For this review, take the finished solid that the model builds, in its own axes (mm). Give positions to 0.01 mm unless a question says otherwise; leave off trailing zeros. Order: outer loops, then holes, each group sorted by start corner. A loop starts at its lowest first (then second) coordinate and runs counter-clockwise, first axis right, second up.
from build123d import *

# Parameters (mm, degrees)
SKETCH1_W           = 48.2
SKETCH1_H           = 18
SKETCH1_R           = 0.6
BOSS_EXTRUDE2_DEPTH = 1.6
SKETCH2_R           = 0.45
CUT_EXTRUDE2_DEPTH  = 1.6
LPATTERN1_COUNT     = 17
LPATTERN1_PITCH     = 2.54
SKETCH3_R           = 0.5
CUT_EXTRUDE4_DEPTH  = 1.6


with BuildPart() as part:
    # Sketch1 → Boss-Extrude2 (new body)
    with BuildSketch(Plane(origin=(0, 0, 0), x_dir=(1, 0, 0), z_dir=(0, 1, 0))):
        with Locations((20.32, 7.62)):
            Rectangle(SKETCH1_W, SKETCH1_H)
        with Locations((-2.54, 0)):
            Circle(SKETCH1_R, mode=Mode.SUBTRACT)
        with Locations((-2.54, 15.24)):
            Circle(SKETCH1_R, mode=Mode.SUBTRACT)
        with Locations((43.18, 15.24)):
            Circle(SKETCH1_R, mode=Mode.SUBTRACT)
        with Locations((43.18, 0)):
            Circle(SKETCH1_R, mode=Mode.SUBTRACT)
    extrude(amount=BOSS_EXTRUDE2_DEPTH)

    # Sketch2 → Cut-Extrude2 (cut)
    with BuildSketch(Plane(origin=(0, 0, 0), x_dir=(1, 0, 0), z_dir=(0, 1, 0))):
        Circle(SKETCH2_R)
        with Locations((0, 15.24)):
            Circle(SKETCH2_R)
    cut_extrude2 = extrude(amount=CUT_EXTRUDE2_DEPTH, mode=Mode.SUBTRACT)

    # LPattern1: Cut-Extrude2 ×17
    with Locations(*[(i * LPATTERN1_PITCH, 0, 0) for i in range(1, LPATTERN1_COUNT)]):
        add(cut_extrude2, mode=Mode.SUBTRACT)

    # Sketch3 → Cut-Extrude4 (cut)
    with BuildSketch(Plane(origin=(0, 0, 0), x_dir=(1, 0, 0), z_dir=(0, 1, 0))):
        with Locations((1.27, 12.7)):
            Circle(SKETCH3_R)
        with Locations((-1.27, 12.7)):
            Circle(SKETCH3_R)
        with Locations((-1.27, 10.16)):
            Circle(SKETCH3_R)
        with Locations((3.81, 12.7)):
            Circle(SKETCH3_R)
        with Locations((3.81, 10.16)):
            Circle(SKETCH3_R)
        with Locations((1.27, 10.16)):
            Circle(SKETCH3_R)
    extrude(amount=CUT_EXTRUDE4_DEPTH, mode=Mode.SUBTRACT)


solid = part.part
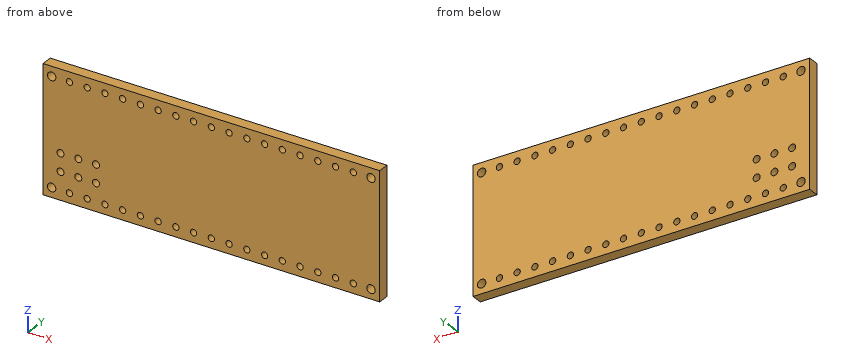
1) To check wall thickness, follow line 1 (Z direction, x = 25.4, y = 1); line 2 (X direction, y = 0.75, z = -12.75); line 3 (Z direction, x = -1, y = 0.5). State the ranges of each line that lie inside material, in increasing order.
Answer sheet:
line 1: z = -16.62 to -15.69, -14.79 to -0.45, 0.45 to 1.38
line 2: x = -3.78 to -1.77, -0.77 to 0.77, 1.77 to 3.31, 4.31 to 44.42
line 3: z = -16.62 to -13.12, -12.28 to -10.58, -9.74 to 1.38
2) We need section B-B on y = 1.2. Count the separate pieces of the cut face and the enclosed holes in it, then the cut area to 3 significant figures.
Answer sheet:
separate pieces: 1
enclosed holes: 44
area: 837 mm2
3) We need section A-A on x = 33.02. Give the boundary of the cut face in (y, z).
Answer sheet:
outline: (0, -16.62) - (1.6, -16.62) - (1.6, -15.69) - (0, -15.69) - close; (0, -14.79) - (1.6, -14.79) - (1.6, -0.45) - (0, -0.45) - close; (0, 0.45) - (1.6, 0.45) - (1.6, 1.38) - (0, 1.38) - close
